Part model, mm, in its own coordinate system. A direction names the side the tool comes from. Coordinates: 2 decimals unless noted, no trailing zeros. Order: outer loops, then holes, each group sorted by start corner. A loop starts at its lowest first (then second) coordinate and runs counter-clockwise, first axis right, second up.
```python
from build123d import *

# Parameters (mm, degrees)
SKETCH1_W                                  = 200
SKETCH1_H                                  = 258
BOSS_EXTRUDE1_DEPTH                        = 10
BOSS_EXTRUDE4_DEPTH                        = 40
SKETCH5_R                                  = 11
CUT_EXTRUDE2_DEPTH                         = 7
SKETCH6_W                                  = 200
SKETCH6_H                                  = 10
BOSS_EXTRUDE6_DEPTH                        = 60
SKETCH7_W                                  = 120
SKETCH7_H                                  = 60
CUT_EXTRUDE3_DEPTH                         = 10
MIRROR4_AT_THE_SECOND_PLANE_COPY_1_SKETC_R = 11
MIRROR4_AT_THE_SECOND_PLANE_COPY_1_DEPTH   = 7
SKETCH8_R                                  = 4
CUT_EXTRUDE4_DEPTH                         = 10
CUT_EXTRUDE6_START                         = -1
SKETCH9_R                                  = 4
CUT_EXTRUDE6_DEPTH                         = 1
SKETCH12_W                                 = 73
SKETCH12_H                                 = 47.27438
SKETCH12_W_2                               = 63
SKETCH12_H_2                               = 37.27438
BOSS_EXTRUDE8_DEPTH                        = 185
SKETCH14_W                                 = 63
SKETCH14_H                                 = 23.684822392
CUT_EXTRUDE7_DEPTH                         = 184
SKETCH15_W                                 = 73
SKETCH15_H                                 = 8
CUT_EXTRUDE8_DEPTH                         = 184
SKETCH16_W                                 = 73
SKETCH16_H                                 = 8
BOSS_EXTRUDE9_DEPTH                        = 47.27
SKETCH17_W                                 = 56.193521686
SKETCH17_H                                 = 1.65349891
CUT_EXTRUDE9_DEPTH                         = 7.27


with BuildPart() as part:
    # Sketch1 → Boss-Extrude1 (new body)
    with BuildSketch(Plane(origin=(0, 0, 0), x_dir=(1, 0, 0), z_dir=(0, 1, 0))):
        Rectangle(SKETCH1_W, SKETCH1_H)
    extrude(amount=BOSS_EXTRUDE1_DEPTH)

    # Sketch2 → Boss-Extrude4 (add)
    with BuildSketch(Plane(origin=(100, 0, 0), x_dir=(0, 0, -1), z_dir=(1, 0, 0))):
        Polygon((89, 0), (89, -50), (99, -50), (129, 0), align=None)
    boss_extrude4 = extrude(amount=-BOSS_EXTRUDE4_DEPTH)

    # Sketch5 → Cut-Extrude2 (cut)
    with BuildSketch(Plane.XY.offset(-89)):
        with Locations((80, -36)):
            Circle(SKETCH5_R)
    cut_extrude2 = extrude(amount=-CUT_EXTRUDE2_DEPTH, mode=Mode.SUBTRACT)

    # Mirror3: Boss-Extrude4, Cut-Extrude2 across plane
    add(boss_extrude4.mirror(Plane(origin=(0, 0, 0), x_dir=(0, 0, 1), z_dir=(1, 0, 0))))
    add(cut_extrude2.mirror(Plane(origin=(0, 0, 0), x_dir=(0, 0, 1), z_dir=(1, 0, 0))), mode=Mode.SUBTRACT)

    # Sketch6 → Boss-Extrude6 (add)
    with BuildSketch(Plane(origin=(0, 10, 0), x_dir=(1, 0, 0), z_dir=(0, 1, 0))):
        with Locations((0, -134)):
            Rectangle(SKETCH6_W, SKETCH6_H)
    extrude(amount=-BOSS_EXTRUDE6_DEPTH)

    # Sketch7 → Cut-Extrude3 (cut)
    with BuildSketch(Plane.XY.offset(139)):
        with Locations((0, -20)):
            Rectangle(SKETCH7_W, SKETCH7_H)
    extrude(amount=-CUT_EXTRUDE3_DEPTH, mode=Mode.SUBTRACT)

    # Mirror4: Cut-Extrude2 across plane
    add(cut_extrude2.mirror(Plane(origin=(0, 0, 0), x_dir=(0, 0, 1), z_dir=(1, 0, 0))), mode=Mode.SUBTRACT)

    # Mirror4 at the second plane: Cut-Extrude2 across plane
    add(cut_extrude2.mirror(Plane.XY.offset(20)), mode=Mode.SUBTRACT)

    # Mirror4 at the second plane copy 1 sketc → Mirror4 at the second plane copy 1 (cut)
    with BuildSketch(Plane(origin=(0, 0, 129), x_dir=(-1, 0, 0), z_dir=(0, 0, -1))):
        with Locations((80, -36)):
            Circle(MIRROR4_AT_THE_SECOND_PLANE_COPY_1_SKETC_R)
    extrude(amount=-MIRROR4_AT_THE_SECOND_PLANE_COPY_1_DEPTH, mode=Mode.SUBTRACT)

    # Sketch8 → Cut-Extrude4 (cut)
    with BuildSketch(Plane(origin=(0, 0, 136), x_dir=(-1, 0, 0), z_dir=(0, 0, -1))):
        with Locations((-80, -36)):
            Circle(SKETCH8_R)
    cut_extrude4 = extrude(amount=-CUT_EXTRUDE4_DEPTH, mode=Mode.SUBTRACT)

    # Mirror5: Cut-Extrude4 across plane
    add(cut_extrude4.mirror(Plane(origin=(0, 0, 0), x_dir=(0, 0, 1), z_dir=(1, 0, 0))), mode=Mode.SUBTRACT)

    # Sketch9 → Cut-Extrude6 (cut)
    with BuildSketch(Plane.XY.offset(-96).offset(CUT_EXTRUDE6_START)):
        with Locations((-80, -36)):
            Circle(SKETCH9_R)
    cut_extrude6 = extrude(amount=CUT_EXTRUDE6_DEPTH, mode=Mode.SUBTRACT)

    # Mirror6: Cut-Extrude6 across plane
    add(cut_extrude6.mirror(Plane(origin=(0, 0, 0), x_dir=(0, 0, 1), z_dir=(1, 0, 0))), mode=Mode.SUBTRACT)

    # Sketch14 → Cut-Extrude7 (cut)
    with BuildSketch(Plane.XY.offset(129)):
        Rectangle(SKETCH14_W, SKETCH14_H)
    extrude(amount=-CUT_EXTRUDE7_DEPTH, mode=Mode.SUBTRACT)

    # Sketch15 → Cut-Extrude8 (cut)
    with BuildSketch(Plane(origin=(0, -17.63719, 0), x_dir=(-1, 0, 0), z_dir=(0, -1, 0))):
        with Locations((0, 59)):
            Rectangle(SKETCH15_W, SKETCH15_H)
    extrude(amount=-CUT_EXTRUDE8_DEPTH, mode=Mode.SUBTRACT)



with BuildPart() as body_2:
    # Sketch12 → Boss-Extrude8 (new body)
    with BuildSketch(Plane.XY.offset(130)):
        with Locations((0, 6)):
            Rectangle(SKETCH12_W, SKETCH12_H)
        with Locations((0, 6)):
            Rectangle(SKETCH12_W_2, SKETCH12_H_2, mode=Mode.SUBTRACT)
    extrude(amount=-BOSS_EXTRUDE8_DEPTH)


with BuildPart() as part_1:
    add(part.part)

    add(body_2.part)  # Boss-Extrude9 merges body 2
    # Sketch16 → Boss-Extrude9 (add)
    with BuildSketch(Plane(origin=(0, -17.63719, 0), x_dir=(-1, 0, 0), z_dir=(0, -1, 0))):
        with Locations((0, 59)):
            Rectangle(SKETCH16_W, SKETCH16_H)
    extrude(amount=-BOSS_EXTRUDE9_DEPTH)

    # Sketch17 → Cut-Extrude9 (cut)
    with BuildSketch(Plane(origin=(0, 29.63719, 0), x_dir=(1, 0, 0), z_dir=(0, 1, 0))):
        with Locations((0, -127.668994325)):
            Rectangle(SKETCH17_W, SKETCH17_H)
    extrude(amount=-CUT_EXTRUDE9_DEPTH, mode=Mode.SUBTRACT)


solid = part_1.part
```
(1) Probe line 1 (Y direction, x = 80, z = 134.5); line 2 (X direction, y = 19.5, z = 66); line 3 (Y direction, x = -80, z = 138). List the from-to ranges inside material, lowest first.
(2) Tool access for faces 1 (the face through (80.521, -32.034, 137.479)), 2 (the face through (80, -19, 129)), 3 (the face through (1, 20, -63)): list every direction of +Z, -Z, +X, -X, +Y, -Y with a clear straight run to the whole face (end or side of a thin tool).
(3) Drop flat-ended pins along their axis: pin 1 (13 mm diameter, centred on x = -80, y = -36, fed in from -Z); pin 2 (1 mm diameter, centred on x = -38, y = 8, fed in from +Z); pin 3 (6.5 mm diameter, centred on x = -81.5, y = -35.5, fed in from -Z). Give the stop position or say it passes through.
(4) Slice it at A-A, the plane y = -3. Give the cut face in (x, z), then the cut area to 3 significant figures.
(5) Slice it at D-D, the plane y = -22. Give the cut face in (x, z).
(6) Slice it at B-B, the plane x = 80. Give the cut face in (y, z).
(7) Slice it at C-C, the plane z = 29. Give the cut face in (x, y), then the cut area to 3 significant figures.
(8) Pull direction X, two halves, no side cores. Call faces 4 (the face through (-80, -50, 134)), 5 (the face through (-80, -36, -97)): +X half, -X half, draft (parallel to the pull), parting line (faces both ways), or undercut.
Here are the results:
1. line 1: y = -50 to -47, -25 to 10
1. line 2: x = -36.5 to -31.5, 31.5 to 36.5
1. line 3: y = -50 to -40, -32 to 10
2. face 1: +Z
2. face 2: +X, -Y
2. face 3: -Z, +X, -X, +Y
3. pin 1: stops at z = -111.3
3. pin 2: stops at z = 129
3. pin 3: stops at z = -109.65
4. outline: (-100, -127.2) - (-60, -127.2) - (-60, -89) - (-100, -89) - close; (-100, 129) - (-60, 129) - (-60, 139) - (-100, 139) - close; (-36.5, -63) - (36.5, -63) - (36.5, 130) - (31.5, 130) - (31.5, -55) - (-31.5, -55) - (-31.5, 130) - (-36.5, 130) - close; (60, -127.2) - (100, -127.2) - (100, -89) - (60, -89) - close; (60, 129) - (100, 129) - (100, 139) - (60, 139) - close
4. area: 6,290 mm2
5. outline: (-100, -115.8) - (-60, -115.8) - (-60, -89) - (-100, -89) - close; (-100, 129) - (-60, 129) - (-60, 139) - (-100, 139) - close; (60, -115.8) - (100, -115.8) - (100, -89) - (60, -89) - close; (60, 129) - (100, 129) - (100, 139) - (60, 139) - close
6. outline: (-50, -99) - (0, -129) - (10, -129) - (10, 139) - (-32, 139) - (-32, 136) - (-25, 136) - (-25, 129) - (0, 129) - (0, -89) - (-25, -89) - (-25, -96) - (-32, -96) - (-32, -97) - (-40, -97) - (-40, -96) - (-47, -96) - (-47, -89) - (-50, -89) - close; (-50, 129) - (-47, 129) - (-47, 136) - (-40, 136) - (-40, 139) - (-50, 139) - close
7. outline: (-100, 0) - (-36.5, 0) - (-36.5, -17.64) - (36.5, -17.64) - (36.5, 0) - (100, 0) - (100, 10) - (36.5, 10) - (36.5, 29.64) - (-36.5, 29.64) - (-36.5, 10) - (-100, 10) - close; hole (-31.5, -12.64) - (31.5, -12.64) - (31.5, 24.64) - (-31.5, 24.64) - close
7. area: 2,370 mm2
8. face 4: draft
8. face 5: undercut
